Geometry: final body of the model. Coordinates: model frame, mm. Face numbers are marked on the shaded views. A direction names the side the tool comes from. Coordinates: 2 decimals unless noted, no trailing zeros. Write each loop counter-clockwise with the first axis right and the second up, starting at its lowest first coordinate (ties: lowest second). Pieces come first, ordered by that corner, then holes.
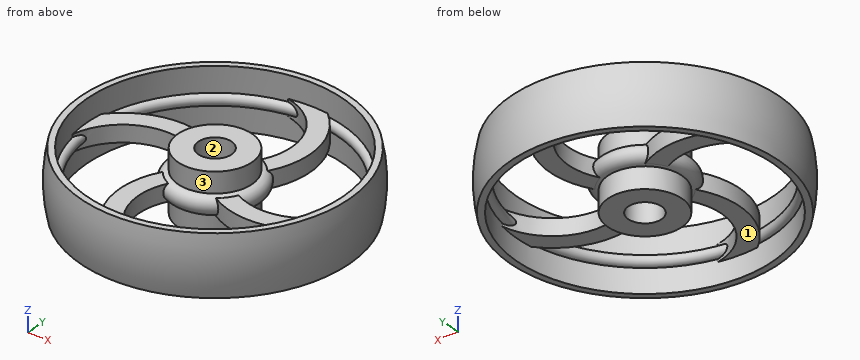
from build123d import *

# Parameters (mm, degrees)
BOSS_EXTRUDE3_DEPTH = 9
CIRPATTERN1_COUNT   = 4


with BuildPart() as part:
    # Sweep1: sweep along a path in Sketch1
    with BuildLine(Plane.XY) as sweep1_path:
        CenterArc((0, 0), 145, 0, 360)
    # Sketch2 → Sweep1 (sweep)
    with BuildSketch(Plane(origin=(0, 0, 0), x_dir=(0, 0, -1), z_dir=(1, 0, 0))):
        with BuildLine():
            Line((5.999166033, 138), (32.050741021, 138))
            Line((32.050741021, 138), (32.050741021, 145))
            ThreePointArc((32.050741021, 145), (-0.460420914, 148.499286236), (-32.949258979, 144.798467992))
            Line((-32.949258979, 144.798467992), (-32.949258979, 138))
            Line((-32.949258979, 138), (-5.999166033, 138))
            ThreePointArc((-5.999166033, 138), (0, 131.899965493), (5.999166033, 138))
        make_face()
    sweep(path=sweep1_path.line)



with BuildPart() as body_2:
    # Sweep2: sweep along a path in Sketch3
    with BuildLine(Plane.XY) as sweep2_path:
        CenterArc((0, 0), 40, 0, 360)
    # Sketch4 → Sweep2 (sweep)
    with BuildSketch(Plane(origin=(0, 0, 0), x_dir=(0, 0, -1), z_dir=(1, 0, 0))):
        with BuildLine():
            Line((-32.5, 40), (-10.449258979, 40))
            ThreePointArc((-10.449258979, 40), (-0.449258979, 50), (9.550741021, 40))
            Line((9.550741021, 40), (32.5, 40))
            Line((32.5, 40), (32.5, 18))
            Line((32.5, 18), (-32.5, 18))
            Line((-32.5, 18), (-32.5, 40))
        make_face()
    sweep(path=sweep2_path.line)


with BuildPart() as part_1:
    add(part.part)

    add(body_2.part)  # Boss-Extrude3 merges body 2
    # Sketch10 → Boss-Extrude3 (add, symmetric)
    with BuildSketch(Plane.XY):
        with BuildLine():
            ThreePointArc((17.330404885, 36.050756809), (23.609351815, 96.881391078), (-23.394040608, 136.002642857))
            ThreePointArc((-23.394040608, 136.002642857), (-2.240713474, 137.981807508), (18.965722986, 136.690531317))
            ThreePointArc((18.965722986, 136.690531317), (47.802187213, 82.535824261), (32.671857062, 23.077039588))
            ThreePointArc((32.671857062, 23.077039588), (25.828973742, 30.542824287), (17.330404885, 36.050756809))
        make_face()
    boss_extrude3 = extrude(amount=BOSS_EXTRUDE3_DEPTH, both=True)

    # CirPattern1: Boss-Extrude3 ×4 about axis
    cirpattern1_axis = Axis((0, 0, 0), (0, 0, 1))
    for i in range(1, CIRPATTERN1_COUNT):
        add(boss_extrude3.rotate(cirpattern1_axis, i * 360 / CIRPATTERN1_COUNT))


solid = part_1.part
Item 1: Material intervals for probe 1 along Y at (x, z) = (0, -23.5); probe 2 along Y at (x, z) = (-34, -15) (3 decimals); probe 3 along Y at (x, z) = (0, -18.5), sorted ascending.
Derived:
probe 1: y = -146.63 to -138, -40 to -18, 18 to 40, 138 to 146.63
probe 2: y = -143.775 to -133.746, -21.071 to 21.071, 133.746 to 143.775
probe 3: y = -147.34 to -138, -40 to -18, 18 to 40, 138 to 147.34
Item 2: Section A-A, the plane z = -27. Output: boundary loops of the cut face in (x, y).
Derived:
outline: circle Ø292.05 at (0, 0); circle Ø80 at (0, 0); hole circle Ø276 at (0, 0); hole circle Ø36 at (0, 0)
Item 3: Pin query (flat end, axial travel): pin 1 (12 mm diameter, centred on x = 53, y = 79, fed in from +Z); pin 2 (4 mm diameter, centred on x = 34.5, z = -10.5, fed in from -Y); pin 3 (10 mm diameter, centred on y = 69, z = -14, fed in from -X). Return the tip coordinate at first contact, or that it passes through.
Derived:
pin 1: stops at z = 9
pin 2: stops at y = -144.54
pin 3: stops at x = -133.32
Item 4: Section B-B, the plane x = 88. State how many separate pieces and enclosed holes the cut face has, plus the area to 3 significant figures.
Derived:
separate pieces: 3
enclosed holes: 0
area: 2,060 mm2
Item 5: Set-up query: the marked faces 1, 2 and 3. Return all of +Z, -Z, +X, -X, +Y, -Y with unobstructed straight access to the full face (end or side cutting, diameter ignored); none if empty.
Derived:
face 1: -Z
face 2: +Z, -Z
face 3: +Z
